Work out the finished part from the listing and answer in its coordinate system (mm). Give positions to 0.01 mm unless a question says otherwise; leave off trailing zeros. Loops run counter-clockwise (first coordinate to the right, second up) from the corner with the lowest first, then second, coordinate; pieces in that order, holes last. Notation, with made-up numbers: M 60,58.5 L 65,58.5 A18 cw 65,91.5 Z; hole C 72,76.25 d6. An arc over 180 degrees is marked long. Use a Markdown table: item, result.
```python
from build123d import *

# Parameters (mm, degrees)
F0_W     = 490
F0_H     = 6
F0_W_2   = 25
F1_DEPTH = 50


# Not quite as in the source:
# - a feature names something its author has since deleted; it is built from what else it names
# - the program builds the solid bodies; features that only make, move or delete a surface that nothing else refers to are left out


with BuildPart() as f1:
    # F0 (on Top) → F1 (new body)
    with BuildSketch(Plane.XY):
        Polygon((0, 1190), (0, 0), (515, 0), (540, 0), (540, 25), (540, 125), (540, 131), (540, 539), (540, 545), (540, 645), (540, 651), (540, 1059), (540, 1065), (540, 1165), (540, 1190), (515, 1190), align=None)
        Polygon((25, 1065), (25, 1165), (515, 1165), (515, 1065), (515, 1059), (515, 651), (515, 645), (515, 545), (515, 539), (515, 131), (515, 125), (515, 25), (25, 25), (25, 125), (25, 131), (25, 539), (25, 545), (25, 645), (25, 651), (25, 1059), align=None, mode=Mode.SUBTRACT)
        Polygon((540, 25), (540, 0), (1030, 0), (1055, 0), (1545, 0), (1570, 0), (1570, 25), (1570, 125), (1570, 131), (1570, 539), (1570, 545), (1570, 645), (1570, 651), (1570, 1059), (1570, 1065), (1570, 1165), (1570, 1190), (1545, 1190), (1055, 1190), (1030, 1190), (540, 1190), (540, 1165), (1030, 1165), (1055, 1165), (1545, 1165), (1545, 1065), (1545, 1059), (1545, 651), (1545, 645), (1545, 545), (1545, 539), (1545, 131), (1545, 125), (1545, 25), (1055, 25), (1030, 25), align=None)
        Polygon((1570, 25), (1570, 0), (2085, 0), (2085, 1190), (1570, 1190), (1570, 1165), (2060, 1165), (2060, 1065), (2060, 1059), (2060, 651), (2060, 645), (2060, 545), (2060, 539), (2060, 131), (2060, 125), (2060, 25), align=None)
        with Locations((270, 542)):
            Rectangle(F0_W, F0_H)
        with Locations((270, 128)):
            Rectangle(F0_W, F0_H)
        with Locations((270, 648)):
            Rectangle(F0_W, F0_H)
        with Locations((270, 1062)):
            Rectangle(F0_W, F0_H)
        with Locations((785, 648)):
            Rectangle(F0_W, F0_H)
        with Locations((1300, 648)):
            Rectangle(F0_W, F0_H)
        with Locations((1300, 542)):
            Rectangle(F0_W, F0_H)
        with Locations((785, 542)):
            Rectangle(F0_W, F0_H)
        with Locations((1815, 542)):
            Rectangle(F0_W, F0_H)
        with Locations((1815, 648)):
            Rectangle(F0_W, F0_H)
        with Locations((1815, 1062)):
            Rectangle(F0_W, F0_H)
        with Locations((1300, 1062)):
            Rectangle(F0_W, F0_H)
        with Locations((785, 1062)):
            Rectangle(F0_W, F0_H)
        with Locations((1815, 128)):
            Rectangle(F0_W, F0_H)
        with Locations((785, 128)):
            Rectangle(F0_W, F0_H)
        with Locations((1300, 128)):
            Rectangle(F0_W, F0_H)
        with Locations((1042.5, 128)):
            Rectangle(F0_W_2, F0_H)
        with Locations((1042.5, 542)):
            Rectangle(F0_W_2, F0_H)
        with Locations((1042.5, 1062)):
            Rectangle(F0_W_2, F0_H)
        with Locations((1042.5, 648)):
            Rectangle(F0_W_2, F0_H)
    extrude(amount=F1_DEPTH)


solid = f1.part
```
(1) A cutting plane is placed at A-A (x = 143). Write down the section's boundary in (y, z).
Entries:
| item | result |
|---|---|
| outline | M 0,0 L 25,0 L 25,50 L 0,50 Z; M 125,0 L 131,0 L 131,50 L 125,50 Z; M 539,0 L 545,0 L 545,50 L 539,50 Z; M 645,0 L 651,0 L 651,50 L 645,50 Z; M 1059,0 L 1065,0 L 1065,50 L 1059,50 Z; M 1165,0 L 1190,0 L 1190,50 L 1165,50 Z |
(2) Given P1, Ø15, axis at y = 602, z = 23, coming from the -X side, flat-ended and moving along its own axis, determine where the tip first touches the part or whether it passes through.
Entries:
| item | result |
|---|---|
| P1 | stops at x = 0 |
(3) The mould has two halves that part along X. Classify faces 1 (the flat face through (1812, 539, 25)), 2 (the flat face through (1037.6, 24.8, 50)): released by +X, released by -X, zero draft, split by the parting line, or undercut.
Entries:
| item | result |
|---|---|
| face 1 | undercut |
| face 2 | zero draft |
(4) A cutting plane is placed at B-B (y = 701). Write down the section's boundary in (x, z), and give its area (3 significant figures).
Entries:
| item | result |
|---|---|
| outline | M 0,0 L 25,0 L 25,50 L 0,50 Z; M 515,0 L 540,0 L 540,50 L 515,50 Z; M 1545,0 L 1570,0 L 1570,50 L 1545,50 Z; M 2060,0 L 2085,0 L 2085,50 L 2060,50 Z |
| area | 5,000 mm² |
(5) A cutting plane is placed at C-C (z = 37.5). Count the separate pieces of the cut face and the enclosed holes in it, and give its area (3 significant figures).
Entries:
| item | result |
|---|---|
| separate pieces | 1 |
| enclosed holes | 15 |
| area | 266,000 mm² |
(6) Consider probe 1 along Y at (x, z) = (692, 30); probe 2 along X at (y, z) = (1007, 41). Determine where each line is inside the solid, lowest interval first. Write a range as [from, to].
Entries:
| item | result |
|---|---|
| probe 1 | y = [0, 25], [125, 131], [539, 545], [645, 651], [1059, 1065], [1165, 1190] |
| probe 2 | x = [0, 25], [515, 540], [1545, 1570], [2060, 2085] |
